Input: dimensioned drawing with shaded views. Units: mm. Origin: part minimum x, y, z. Give positions to 0.01 mm unless a question says otherwise; leave off trailing zeros. Write each loop counter-clockwise with the first axis right and the second up, starting at its lowest first coordinate (ties: lowest second). Pieces come first, ordered by that corner, then holes.
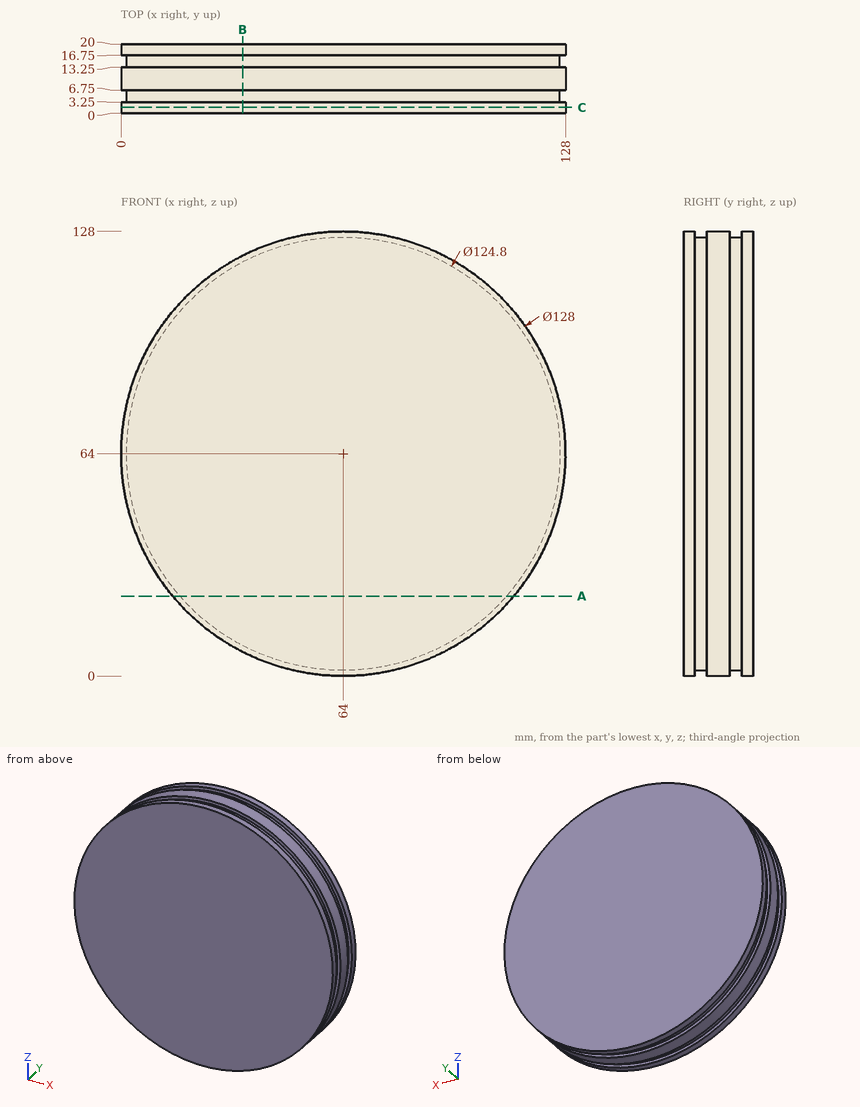
1. Line query: L1, parallel to Y at x = 118, z = 30; L2, parallel to Z at x = 114, y = 13.5; L3, parallel to Z at x = 16.5, y = 5.75. Output: solid intervals per line, ascending.
2. Cut plane C-C, the plane y = 1.75. Return the cut outline in (x, z), then the cut area to 3 significant figures.
3. Contact query for flat-ended pins moving along their axis: P1, Ø1, axis at y = 15.5, z = 75, coming from the -X side; P2, Ø6, axis at x = 52, y = 2.5, coming from the +Z side; P3, Ø1, axis at y = 2.5, z = 44, coming from the -X side; P4, Ø6, axis at x = 107.5, z = 31, coming from the -Y side. Output: stop coordinate, or through.
4. Cut plane B-B, the plane x = 35. Return the cut outline in (y, z).
5. Cut plane A-A, the plane z = 23. Return the cut outline in (x, y), then the cut area to 3 significant figures.
Response values:
1. L1: y = 0 to 3.25, 6.75 to 13.25, 16.75 to 20
1. L2: z = 26.67 to 101.33
1. L3: z = 23.53 to 104.47
2. outline: circle Ø128 at (64, 64)
2. area: 12,900 mm2
3. P1: stops at x = 2.49
3. P2: stops at z = 127.36
3. P3: stops at x = 3.04
3. P4: stops at y = 0
4. outline: (0, 6.95) - (3.25, 6.95) - (3.25, 8.75) - (6.75, 8.75) - (6.75, 6.95) - (13.25, 6.95) - (13.25, 8.75) - (16.75, 8.75) - (16.75, 6.95) - (20, 6.95) - (20, 121.05) - (16.75, 121.05) - (16.75, 119.25) - (13.25, 119.25) - (13.25, 121.05) - (6.75, 121.05) - (6.75, 119.25) - (3.25, 119.25) - (3.25, 121.05) - (0, 121.05) - close
5. outline: (14.86, 0) - (113.14, 0) - (113.14, 3.25) - (111.04, 3.25) - (111.04, 6.75) - (113.14, 6.75) - (113.14, 13.25) - (111.04, 13.25) - (111.04, 16.75) - (113.14, 16.75) - (113.14, 20) - (14.86, 20) - (14.86, 16.75) - (16.96, 16.75) - (16.96, 13.25) - (14.86, 13.25) - (14.86, 6.75) - (16.96, 6.75) - (16.96, 3.25) - (14.86, 3.25) - close
5. area: 1,940 mm2
